Read the model definition and answer for the solid it produces. Units are mm, in the model's axes. A direction names the side the tool comes from. Round coordinates to 2 decimals unless told otherwise and drop trailing zeros. Order: outer loops, then holes, each group sorted by start corner. A loop starts at its lowest first (then second) coordinate and runs counter-clockwise, first axis right, second up. Notation, with made-up numbers: (-35, 52.5) - (2, 52.5) arc R19 ccw to (2, 78.5) - close; hole circle Ø5 at (-14.75, -23). An arc over 180 degrees is marked (long way). Answer as a JSON object with one key per item and string values. Group by question number.
Q1. A tool of negligible diameter and unlimited length cuts with its end or side. For faces 1 (the flat face through (-6, 0, 0)), 2 (the flat face through (1.18, 9.59, 0.11)), 3 (the flat face through (-14.5, -12.5, 0.1)), from which of +Z, -Z, +X, -X, +Y, -Y can it reach the whole face along a straight path? Write none if from no direction.
Q2. Given pin 1 Ø7.5 at (y, z) = (-5, 0) entering from +X; pin 2 Ø0.8 at (x, z) = (-14.5, -2.5) entering from -Y; pin 3 Ø8 at (x, z) = (-5.5, 3.5) entering from +Y, each flat-ended and moving along its own axis, determine where each tip first touches the part or whether it passes through.
Q3. A cutting plane is placed at A-A on y = -6. Determine the outline of the cut face in (x, z).
Q4. The mould has two halves that part along Z. Classify faces 4 (the flat face through (2, -2, 7.5)), 5 (the flat face through (2, -2, -7.5)), 6 (the flat face through (0, -7, 0)), 7 (the flat face through (-11, 3.6, 0.1)): pulls with the +Z half, pulls with the -Z half, needs draft (parallel to the pull), parting line crosses it, or undercut.
Q5. Consider line 1 (Y direction, x = 5, z = -1.25); line 2 (Y direction, x = 7, z = 5); line 3 (Y direction, x = 2.5, z = 3). Determine where each line is inside the solid, lowest interval first.
```python
from build123d import *

# Parameters (mm, degrees)
F1_DEPTH    = 7.5
F2_T1_DEPTH = 40.8093190584
F2_T3_DEPTH = 25.3553390593
F2_T5_DEPTH = 40
F2_T7_DEPTH = 29.3169174454
F3_R        = 1
F5_DEPTH    = 1
F7_R        = 2


# Not quite as in the source:
# - a fillet or chamfer that OpenCascade refuses, or shapes differently, is made with other operations: its cross-section is extruded or revolved along the edge and cut away or added


with BuildPart() as f1:
    # F0 (on Top) → F1 (new body, symmetric)
    with BuildSketch(Plane.XY):
        with BuildLine():
            Line((12, 11.4339222498), (12, 7.4339222498))
            Line((12, 7.4339222498), (21.3969262079, 10.8541236831))
            Line((21.3969262079, 10.8541236831), (21.3969262079, 14.4325955519))
            Line((21.3969262079, 14.4325955519), (3.5841766184, 12.5604001283))
            Line((3.5841766184, 12.5604001283), (0.0437047985, 8.1882815452))
            Line((0.0437047985, 8.1882815452), (-8, 7.3428541036))
            Line((-8, 7.3428541036), (-12.3721185831, 10.8833259234))
            Line((-12.3721185831, 10.8833259234), (-16, 10.5020202215))
            Line((-16, 10.5020202215), (-16, -1.5))
            Line((-16, -1.5), (-14, -1.5))
            Line((-14, -1.5), (-11, 0))
            Line((-11, 0), (0, 0))
            Line((0, 0), (0, -14))
            Line((0, -14), (-11, -14))
            Line((-11, -14), (-14, -12.5))
            Line((-14, -12.5), (-16, -12.5))
            Line((-16, -12.5), (-16, -19))
            Line((-16, -19), (13.1190956366, -19))
            ThreePointArc((13.1190956366, -19), (16.1198863152, -4.0924328046), (2.9233065352, 3.4633984857))
            Line((2.9233065352, 3.4633984857), (-11, 2))
            Line((-11, 2), (-11, 5.0165248387))
            Line((-11, 5.0165248387), (7, 6.9084010735))
            Line((7, 6.9084010735), (6.5841766184, 10.8646962749))
            Line((6.5841766184, 10.8646962749), (12, 11.4339222498))
        make_face()
        with BuildLine():
            ThreePointArc((3, 0.4520743715), (13.0884587778, -4.7273070645), (11.8517750862, -16))
            Line((11.8517750862, -16), (3, -16))
            Line((3, -16), (3, 0.4520743715))
        make_face(mode=Mode.SUBTRACT)
    extrude(amount=F1_DEPTH, both=True)

    # F2: fillet of radius 5 on 4 edges, made by hand

    # F2_s2 → F2_t1 (cut)
    with BuildSketch(Plane.XY.offset(-20.4046595292)):
        with BuildLine():
            ThreePointArc((16.2633396262, 13.89303386), (19.3329992123, 13.2230634603), (21.3969262079, 10.8541236831))
            Line((21.3969262079, 10.8541236831), (21.3969262079, 14.4325955519))
            Line((21.3969262079, 14.4325955519), (16.2633396262, 13.89303386))
        make_face()
    extrude(amount=F2_T1_DEPTH, mode=Mode.SUBTRACT)

    # F2_s4 → F2_t3 (cut)
    with BuildSketch(Plane.XY.offset(-12.6776695297)):
        with BuildLine():
            ThreePointArc((2.2808114131, 10.9508781424), (3.7807474191, 12.1983617504), (5.6438989041, 12.776885664))
            Line((5.6438989041, 12.776885664), (3.5841766184, 12.5604001283))
            Line((3.5841766184, 12.5604001283), (2.2808114131, 10.9508781424))
        make_face()
    extrude(amount=F2_T3_DEPTH, mode=Mode.SUBTRACT)

    # F2_s6 → F2_t5 (cut)
    with BuildSketch(Plane.XY.offset(-20)):
        with BuildLine():
            ThreePointArc((-11, -19), (-14.5355339059, -17.5355339059), (-16, -14))
            Line((-16, -14), (-16, -19))
            Line((-16, -19), (-11, -19))
        make_face()
    extrude(amount=F2_T5_DEPTH, mode=Mode.SUBTRACT)

    # F2_s8 → F2_t7 (cut)
    with BuildSketch(Plane.XY.offset(-14.6584587227)):
        with BuildLine():
            ThreePointArc((14.9920579896, -16.8341336537), (13.1998162834, -18.4255320736), (10.8728728234, -19))
            Line((10.8728728234, -19), (13.1190956366, -19))
            ThreePointArc((13.1190956366, -19), (14.115390519, -17.9687915418), (14.9920579896, -16.8341336537))
        make_face()
    extrude(amount=F2_T7_DEPTH, mode=Mode.SUBTRACT)

    # F3
    f3_edges = [f1.edges().sort_by_distance(p)[0] for p in [
        (21.396926, 10.854124, 0),
        (7, 6.908401, 0),
        (-11, 5.016525, 0),
        (-11, 2, 0),
        (12, 11.433922, 0),
        (6.584177, 10.864696, 0),
        (0, 0, 0),
        (0, -14, 0),
        (11.851775, -16, 0),
        (3, -16, 0),
        (3, 0.452074, 0),
        (-16, -12.5, 0),
        (-16, -1.5, 0),
    ]]
    fillet(f3_edges, radius=F3_R)

    # F4 (on face) → F5 (join)
    with BuildSketch(Plane.XY.offset(7.5)):
        with BuildLine():
            Line((-5.9013941166, 5.552409911), (-10.1045284633, 5.1106426898))
            ThreePointArc((-10.1045284633, 5.1106426898), (-10.7431448255, 4.7852514008), (-11, 4.1161207944))
            Line((-11, 4.1161207944), (-11, 3.1106125148))
            ThreePointArc((-11, 3.1106125148), (-10.6691306064, 2.3674676894), (-9.8954715367, 2.1160906195))
            Line((-9.8954715367, 2.1160906195), (-5.5878087268, 2.5688442249))
            Line((-5.5878087268, 2.5688442249), (-5.9013941166, 5.552409911))
        make_face()
    extrude(amount=-F5_DEPTH)

    # F6: F1 across plane


with BuildPart() as f1_1:
    add(f1.part)
    add(f1.part.mirror(Plane.XY))

    # F7
    f7_edges = [f1_1.edges().sort_by_distance(p)[0] for p in [
        (-12.372119, 10.883326, 0),
        (-16, 10.50202, 0),
    ]]
    fillet(f7_edges, radius=F7_R)


solid = f1_1.part
```
Result set:
{
 "1": {"face 1": "+Z, -Z", "face 2": "+Z, -Z, +Y", "face 3": "+Z, -Z, -X"},
 "2": {"pin 1": "stops at x = 17.26", "pin 2": "stops at y = -17.92", "pin 3": "stops at y = 8.56"},
 "3": {"outline": "(0, -7.5) - (3, -7.5) - (3, 7.5) - (0, 7.5) - close; (13.66, -7.5) - (16.81, -7.5) - (16.81, 7.5) - (13.66, 7.5) - close"},
 "4": {"face 4": "pulls with the +Z half", "face 5": "pulls with the -Z half", "face 6": "needs draft", "face 7": "undercut"},
 "5": {"line 1": "y = -19 to -16, 0.51 to 3.51, 6.7 to 12.67", "line 2": "y = -19 to -16, 0.16 to 3.25, 10.7 to 12.92", "line 3": "y = -19 to 3.42, 6.44 to 11.2"}
}
